from build123d import *

# Parameters (mm, degrees)
SKETCH1_R           = 63.5
SKETCH1_R_2         = 55.372
BOSS_EXTRUDE1_DEPTH = 3.175
BOSS_EXTRUDE2_DEPTH = 3.175
SKETCH37_R          = 0.889
CUT_EXTRUDE19_DEPTH = 136.856626854
CIRPATTERN7_COUNT   = 7


with BuildPart() as part:
    # Sketch1 → Boss-Extrude1 (new body)
    with BuildSketch(Plane(origin=(0, 0, 0), x_dir=(1, 0, 0), z_dir=(0, 1, 0))):
        with Locations(Location((0, 0, 0), (0, 0, 270))):
            Circle(SKETCH1_R)
        with Locations(Location((0, 0, 0), (0, 0, 270))):
            Circle(SKETCH1_R_2, mode=Mode.SUBTRACT)
    extrude(amount=BOSS_EXTRUDE1_DEPTH)

    # Sketch2 → Boss-Extrude2 (add)
    with BuildSketch(Plane(origin=(0, 0, 0), x_dir=(1, 0, 0), z_dir=(0, 1, 0))):
        with BuildLine():
            ThreePointArc((63.3815597, 3.87658226), (63.5, 0), (63.3815597, -3.87658226))
            ThreePointArc((63.3815597, -3.87658226), (80.090490582, -1.128517213), (96.339970744, -5.892405036))
            ThreePointArc((96.339970744, -5.892405036), (96.52, 0), (96.339970744, 5.892405036))
            ThreePointArc((96.339970744, 5.892405036), (80.090490582, 1.128517213), (63.3815597, 3.87658226))
        make_face()
        with BuildLine():
            ThreePointArc((-8.955065497, 62.865386358), (-15.008770651, 78.67971172), (-13.611699556, 95.555387264))
            ThreePointArc((-13.611699556, 95.555387264), (-21.477720545, 94.100042084), (-29.19621118, 91.998324184))
            ThreePointArc((-29.19621118, 91.998324184), (-20.615412412, 77.400032324), (-19.208033671, 60.525213279))
            ThreePointArc((-19.208033671, 60.525213279), (-14.130079306, 61.907922424), (-8.955065497, 62.865386358))
        make_face()
        with BuildLine():
            ThreePointArc((64.985862756, -71.364893623), (51.087579034, -61.691324359), (42.753857076, -46.95058791))
            ThreePointArc((42.753857076, -46.95058791), (39.591602418, -49.646299137), (36.25981044, -52.129417289))
            ThreePointArc((36.25981044, -52.129417289), (48.776538257, -63.53431788), (55.114911869, -79.236714279))
            ThreePointArc((55.114911869, -79.236714279), (60.179235675, -75.462374688), (64.985862756, -71.364893623))
        make_face()
        with BuildLine():
            ThreePointArc((-14.861314783, -95.36902916), (-16.037370419, -78.4765123), (-9.777180778, -62.742782342))
            ThreePointArc((-9.777180778, -62.742782342), (-14.130079306, -61.907922424), (-18.414137508, -60.77145333))
            ThreePointArc((-18.414137508, -60.77145333), (-19.600511119, -77.663248687), (-27.989489013, -92.372609061))
            ThreePointArc((-27.989489013, -92.372609061), (-21.477720545, -94.100042084), (-14.861314783, -95.36902916))
        make_face()
        with BuildLine():
            ThreePointArc((-83.618837729, -48.207887082), (-71.195081366, -36.701779549), (-55.012393243, -31.715715185))
            ThreePointArc((-55.012393243, -31.715715185), (-57.211523112, -27.551617434), (-59.096010784, -23.235995986))
            ThreePointArc((-59.096010784, -23.235995986), (-73.084013888, -32.77937075), (-89.825936391, -35.318713899))
            ThreePointArc((-89.825936391, -35.318713899), (-86.96151513, -41.8784585), (-83.618837729, -48.207887082))
        make_face()
        with BuildLine():
            ThreePointArc((-89.979187785, 34.926439348), (-73.226344714, 32.460170557), (-59.196834069, 22.977920624))
            ThreePointArc((-59.196834069, 22.977920624), (-57.211523112, 27.551617434), (-54.87348409, 31.955449361))
            ThreePointArc((-54.87348409, 31.955449361), (-71.034262424, 37.012076334), (-83.407695816, 48.572283029))
            ThreePointArc((-83.407695816, 48.572283029), (-86.96151513, 41.8784585), (-89.979187785, 34.926439348))
        make_face()
        with BuildLine():
            ThreePointArc((53.3732562, 80.420183553), (47.378936921, 64.583253007), (35.113984342, 52.908015495))
            ThreePointArc((35.113984342, 52.908015495), (39.591602418, 49.646299137), (43.767904494, 46.006744465))
            ThreePointArc((43.767904494, 46.006744465), (52.421210722, 60.562173831), (66.52721483, 69.930251586))
            ThreePointArc((66.52721483, 69.930251586), (60.179235675, 75.462374688), (53.3732562, 80.420183553))
        make_face()
    extrude(amount=BOSS_EXTRUDE2_DEPTH)

    # Sketch37 → Cut-Extrude19 (cut, through all)
    with BuildSketch(Plane(origin=(0, 3.175, 0), x_dir=(1, 0, 0), z_dir=(0, 1, 0))):
        with Locations(Location((91.44, 0, 0), (0, 0, 270))):
            Circle(SKETCH37_R)
    cut_extrude19 = extrude(amount=-CUT_EXTRUDE19_DEPTH, mode=Mode.SUBTRACT)

    # CirPattern7: Cut-Extrude19 ×7 about axis
    cirpattern7_axis = Axis((0, 0, 0), (0, 1, 0))
    for i in range(1, CIRPATTERN7_COUNT):
        add(cut_extrude19.rotate(cirpattern7_axis, i * 360 / CIRPATTERN7_COUNT), mode=Mode.SUBTRACT)


solid = part.part
Build history of the part. All positions in model axes, mm. A direction names the side the tool comes from. Give positions to 0.01 mm unless a question says otherwise; leave off trailing zeros. Order: outer loops, then holes, each group sorted by start corner. A loop starts at its lowest first (then second) coordinate and runs counter-clockwise, first axis right, second up. Notation, with made-up numbers: M -1.5,0 L 29.5,0 A15 cw 29.5,25 Z; hole C 28.5,-17 d3. An arc over 180 degrees is marked long. Put each result on its own line as item: value.
Item 1: Cut at D-D on y = 2.55. Count the separate pieces of the cut face and the enclosed holes in it, then the cut area to 3 significant figures.
Results are:
separate pieces: 1
enclosed holes: 8
area: 4,590 mm2
Item 2: Which spindle directions (+Z, -Z, +X, -X, +Y, -Y) get a long thin tool onto all of the face, cutting with end or side? Do faces 1 (the face through (51.25, 1.57, 61.87)), 2 (the face through (48.64, 1.57, 63.34)), 3 (the face through (-14.974, 1.565, -78.443)), 4 (the face through (47.51, 1.57, -64.78)). Say none if no direction does.
Results are:
face 1: +X, +Y, -Y
face 2: +Z, +Y, -Y
face 3: +Y, -Y
face 4: -Z, +Y, -Y
Item 3: Cut at C-C on x = 60.5. Write the cut outline in (y, z) (3 decimals), then the cut area to 3 significant figures.
Results are:
outline: M 0,-75.205 L 3.175,-75.205 L 3.175,-67.018 L 0,-67.018 Z; M 0,-19.287 L 3.175,-19.287 L 3.175,19.287 L 0,19.287 Z; M 0,69.201 L 3.175,69.201 L 3.175,75.205 L 0,75.205 Z
area: 168 mm2
Item 4: Cut at A-A on x = 0. Write the cut outline in (y, z) (3 decimals), then the cut area to 3 significant figures.
Results are:
outline: M 0,-63.5 L 3.175,-63.5 L 3.175,-55.372 L 0,-55.372 Z; M 0,55.372 L 3.175,55.372 L 3.175,63.5 L 0,63.5 Z
area: 51.6 mm2
Item 5: Wall check: probe 1 along X at (y, z) = (2.45, 44); probe 2 along Z at (x, y) = (47, 1.95); probe 3 along X at (y, z) = (1.1, -4.5). Give the ranges that are in metal, low to high.
Results are:
probe 1: -85.91 to -80.28, -45.78 to -33.62, 33.62 to 45.78
probe 2: -64.02 to -53.3, -42.7 to -29.28, 29.28 to 42.7, 56.31 to 61.18
probe 3: -63.34 to -55.19, 55.19 to 63.34, 93.59 to 96.42
Item 6: Drop a flat-ended pin along its axis: pin 1 Ø1.6 at (x, z) = (-20.35, -89.15) entering from +Y. Give the stop position or say it passes through.
Results are:
pin 1: through
Item 7: Cut at B-B on z = 14. Write the cut outline in (x, y) (3 decimals), then the cut area to 3 significant figures.
Results are:
outline: M -61.937,0 L -53.573,0 L -53.573,3.175 L -61.937,3.175 Z; M 53.573,0 L 61.937,0 L 61.937,3.175 L 53.573,3.175 Z
area: 53.1 mm2
Item 8: Pull direction Z, two halves, no side cores. Call faces 5 (the face through (57.707, 1.565, -26.498)), 6 (the face through (46.69, 1.57, 29.77)), 7 (the face through (13.935, 1.565, 61.952)), 8 (the face through (-38, 3.175, -43)): +Z half, -Z half, draft (parallel to the pull), parting line (faces both ways), or undercut.
Results are:
face 5: undercut
face 6: undercut
face 7: +Z half
face 8: draft
